Build history of the part. All positions in model axes, mm. A direction names the side the tool comes from. Coordinates: 2 decimals unless noted, no trailing zeros. Loops run counter-clockwise (first coordinate to the right, second up) from the corner with the lowest first, then second, coordinate; pieces in that order, holes last. Notation, with made-up numbers: M -1,63.5 L 29,63.5 A9 ccw 29,77.5 Z; hole C 57,47.5 d6. An arc over 180 degrees is marked long. Write each question's results on one line, items separated by ' | '. Start each with the question number.
from build123d import *

# Parameters (mm, degrees)
SKETCH_1_W          = 24.73
SKETCH_1_H          = 45.23
EXTRUDE_1_DEPTH     = 32
CHAMFER_1_SIZE      = 2
EXTRUDE_2_DEPTH     = 1
SKETCH_3_R          = 1
CUT_EXTRUDE_1_DEPTH = 4
SKETCH_4_R          = 9.975
EXTRUDE_3_DEPTH     = 3
SKETCH_5_R          = 2
SKETCH_5_R_2        = 1
CUT_EXTRUDE_2_DEPTH = 3
SKETCH_6_W          = 20.33
SKETCH_6_H          = 12
EXTRUDE_4_DEPTH     = 2
CHAMFER_2_SIZE      = 2
SKETCH_7_W          = 22.33
SKETCH_7_H          = 5
CUT_EXTRUDE_3_DEPTH = 2
SKETCH_8_R          = 3
EXTRUDE_5_DEPTH     = 4.1
CUT_EXTRUDE_START   = -4
SKETCH_9_R          = 1
CUT_EXTRUDE_4_DEPTH = 4
FILLET_1_R          = 1


with BuildPart() as part:
    # 스케치1 → 보스-돌출1 (new body)
    with BuildSketch(Plane.XY):
        Rectangle(SKETCH_1_W, SKETCH_1_H)
    extrude(amount=EXTRUDE_1_DEPTH)

    # 모따기1
    chamfer_1_edges = [part.edges().sort_by_distance(p)[0] for p in [
        (-12.365, 22.615, 16),
        (12.365, 22.615, 16),
    ]]
    chamfer(chamfer_1_edges, length=CHAMFER_1_SIZE)

    # 스케치2 → 보스-돌출2 (add)
    with BuildSketch(Plane.XY.offset(32)):
        with BuildLine():
            Line((-7, -22.615), (7, -22.615))
            Line((7, -22.615), (7, 2.753205655))
            ThreePointArc((7, 2.753205655), (0, 0.5), (-7, 2.753205655))
            Line((-7, 2.753205655), (-7, -22.615))
        make_face()
    extrude(amount=EXTRUDE_2_DEPTH)

    # 스케치3 → 컷-돌출1 (cut)
    with BuildSketch(Plane.XY.offset(32)):
        with Locations((-10.25, 3.885)):
            Circle(SKETCH_3_R)
        with Locations((-10.25, -16.615)):
            Circle(SKETCH_3_R)
        with Locations((10.25, -16.615)):
            Circle(SKETCH_3_R)
        with Locations((10.25, 3.885)):
            Circle(SKETCH_3_R)
    extrude(amount=-CUT_EXTRUDE_1_DEPTH, mode=Mode.SUBTRACT)

    # 스케치4 → 보스-돌출3 (add)
    with BuildSketch(Plane.XY.offset(32)):
        with Locations((0, 12.5)):
            Circle(SKETCH_4_R)
    extrude(amount=EXTRUDE_3_DEPTH)

    # 스케치5 → 컷-돌출2 (cut)
    with BuildSketch(Plane.XY.offset(35)):
        with Locations((0, 12.5)):
            Circle(SKETCH_5_R)
        with Locations((0, 19.5)):
            Circle(SKETCH_5_R_2)
        with Locations((7, 12.5)):
            Circle(SKETCH_5_R_2)
        with Locations((0, 5.5)):
            Circle(SKETCH_5_R_2)
        with Locations((-7, 12.5)):
            Circle(SKETCH_5_R_2)
    extrude(amount=-CUT_EXTRUDE_2_DEPTH, mode=Mode.SUBTRACT)

    # 스케치6 → 보스-돌출4 (add)
    with BuildSketch(Plane(origin=(0, 0, 0), x_dir=(-1, 0, 0), z_dir=(0, 0, -1))):
        with Locations((0, -12.115)):
            Rectangle(SKETCH_6_W, SKETCH_6_H)
    extrude(amount=EXTRUDE_4_DEPTH)

    # 모따기2
    chamfer_2_edges = [part.edges().sort_by_distance(p)[0] for p in [
        (0, -6.115, -2),
    ]]
    chamfer(chamfer_2_edges, length=CHAMFER_2_SIZE - 0.0001)  # a hair under: the kernel refuses the full size

    # 스케치7 → 컷-돌출3 (cut)
    with BuildSketch(Plane(origin=(0, 0, 0), x_dir=(-1, 0, 0), z_dir=(0, 0, -1))):
        with Locations((0, -3.615)):
            Rectangle(SKETCH_7_W, SKETCH_7_H)
    extrude(amount=-CUT_EXTRUDE_3_DEPTH, mode=Mode.SUBTRACT)

    # 스케치8 → 보스-돌출5 (add)
    with BuildSketch(Plane(origin=(0, 0, 0), x_dir=(-1, 0, 0), z_dir=(0, 0, -1))):
        with Locations(Location((0, 12.5, 0), (0, 0, 180))):
            Circle(SKETCH_8_R)
    extrude(amount=EXTRUDE_5_DEPTH)

    # 스케치9 → 컷-돌출4 (cut)
    with BuildSketch(Plane(origin=(0, 0, 0), x_dir=(-1, 0, 0), z_dir=(0, 0, -1)).offset(CUT_EXTRUDE_START)):
        with Locations(Location((-10.25, 3.885, 0), (0, 0, 180))):
            Circle(SKETCH_9_R)
        with Locations(Location((10.25, 3.885, 0), (0, 0, 180))):
            Circle(SKETCH_9_R)
        with Locations((-10.25, -20.615)):
            Circle(SKETCH_9_R)
        with Locations((10.25, -20.615)):
            Circle(SKETCH_9_R)
    extrude(amount=CUT_EXTRUDE_4_DEPTH, mode=Mode.SUBTRACT)

    # 필렛1
    fillet_1_edges = [part.edges().sort_by_distance(p)[0] for p in [
        (12.365, -22.615, 16),
        (-12.365, -22.615, 16),
    ]]
    fillet(fillet_1_edges, radius=FILLET_1_R)


solid = part.part
1. Pin check, flat tips, straight feed: pin 1 (1 mm diameter, centred on x = 1, z = -1, fed in from -Y) (3 decimals); pin 2 (1.2 mm diameter, centred on x = -10.25, y = -20.615, fed in from +Z); pin 3 (4 mm diameter, centred on x = 6.5, y = -17.5, fed in from +Z). Stop position of each tip, or through.
2. Wall check: line 1 along Y through (x, z) = (-10.25, 2.75) (3 decimals); line 2 along Y through (x, z) = (-10.25, 30.65) (3 decimals); line 3 along Y through (x, z) = (0, 33.2) (3 decimals). Give the ranges that are in metal, low to high.
3. Band-saw the part on D-D, the plane y = 2. List the corners of the cut face in (x, z) (3 decimals).
4. Band-saw the part on C-C, the plane x = 4. List the corners of the cut face in (y, z) (3 decimals), plus the area to 3 significant figures.
5. Band-saw the part on A-A, the plane y = -5. List the corners of the cut face in (x, z) (3 decimals), plus the area to 3 significant figures.
6. Which spindle directions (+Z, -Z, +X, -X, +Y, -Y) get a long thin tool onto all of the face, cutting with end or side? Do faces 1 (the flat face through (-10, -17, 28)), 2 (the flat face through (-7, -9.8, 32.5)), 3 (the flat face through (-10.165, -12, -1)), 4 (the flat face through (0, -1.115, 1)). Say none if no direction does.
7. Band-saw the part on B-B, the plane x = -4.75. List the corners of the cut face in (y, z) (3 decimals), plus the area to 3 significant figures.
Checked values:
1) pin 1: y = -18.115 | pin 2: z = 32 | pin 3: z = 33
2) line 1: -22.615 to -21.615, -19.615 to 2.885, 4.885 to 22.615 | line 2: -22.615 to -17.615, -15.615 to 2.885, 4.885 to 22.615 | line 3: 2.525 to 4.5, 6.5 to 10.5, 14.5 to 18.5, 20.5 to 22.475
3) outline: M -12.365,0 L 12.365,0 L 12.365,32 L 7,32 L 7,33 L 5.809,33 L 5.809,32 L -5.809,32 L -5.809,33 L -7,33 L -7,32 L -12.365,32 Z
4) outline: M -22.615,0 L -18.115,0 L -18.115,-2 L -8.115,-2 L -6.115,0 L -6.115,2 L -1.115,2 L -1.115,0 L 22.615,0 L 22.615,32 L 21.638,32 L 21.638,35 L 3.362,35 L 3.362,32 L 1.186,32 L 1.186,33 L -22.615,33 Z | area: 1,540 mm²
5) outline: M -12.365,0 L -11.165,0 L -11.165,2 L 11.165,2 L 11.165,0 L 12.365,0 L 12.365,32 L 7,32 L 7,33 L -7,33 L -7,32 L -12.365,32 Z | area: 761 mm²
6) face 1: +Z | face 2: +Z, -X, -Y | face 3: -Z, -X, +Y, -Y | face 4: -Z
7) outline: M -22.615,0 L -18.115,0 L -18.115,-2 L -8.115,-2 L -6.115,0 L -6.115,2 L -1.115,2 L -1.115,0 L 22.615,0 L 22.615,32 L 21.271,32 L 21.271,35 L 3.729,35 L 3.729,32 L 1.48,32 L 1.48,33 L -22.615,33 Z | area: 1,540 mm²
